For this review, use the dimensioned drawing (mm, ordinates from the lowest corner) and the shaded views. Coordinates: 2 decimals unless noted, no trailing zeros. Loops run counter-clockwise (first coordinate to the right, second up) from the corner with the lowest first, then second, coordinate; pieces in that order, holes last. Notation, with made-up numbers: M 20,-23.5 L 77,-23.5 A25 cw 77,6.5 Z; hole C 34.25,-15 d8. An arc over 180 degrees is marked long. Write item = value, one per line. Start each with the question number.
Q1. Wall thickness on probe 1 along Y at (x, z) = (4, 30); probe 2 along Y at (x, z) = (1.25, 26); probe 3 along Z at (x, y) = (1.75, 31.5): over which ranges is each line inside the solid? List them lowest first.
Q2. We need section C-C on z = 30. Give the boundary of the cut face in (x, y).
Q3. We need section B-B on x = 4.75. Give the boundary of the cut face in (y, z), and give its area (3 significant figures).
Q4. We need section A-A on y = 25. Give the boundary of the cut face in (x, z).
Q5. Clearance check with a flat-ended pin moving along its axis: pin 1 Ø5 at (y, z) = (38.5, 93) entering from -X. State where the tip first meets the part, or that it passes through.
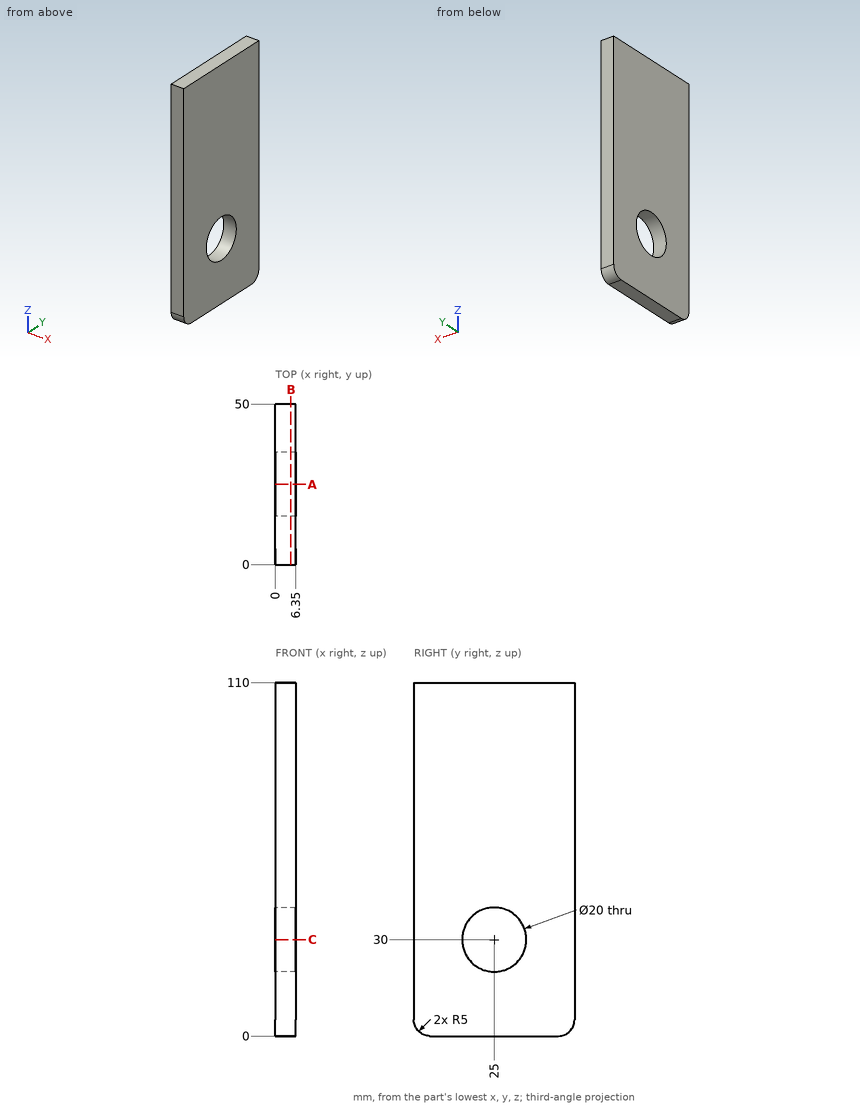
Returned:
q1.probe_1 = 0 to 15, 35 to 50
q1.probe_2 = 0 to 15.83, 34.17 to 50
q1.probe_3 = 0 to 22.4, 37.6 to 110
q2.outline = M 0,0 L 6.35,0 L 6.35,15 L 0,15 Z; M 0,35 L 6.35,35 L 6.35,50 L 0,50 Z
q3.outline = M 0,5 A5 ccw 5,0 L 45,0 A5 ccw 50,5 L 50,110 L 0,110 Z; hole C 25,30 d20
q3.area = 5,180 mm^2
q4.outline = M 0,0 L 6.35,0 L 6.35,20 L 0,20 Z; M 0,40 L 6.35,40 L 6.35,110 L 0,110 Z
q5.pin_1 = 0
